Autodesk Inventor part; units mm, degrees
ref_plane "YZ Plane" through (0, 0, 0) normal (1, 0, 0) x (0, 1, 0)
ref_plane "XZ Plane" through (0, 0, 0) normal (0, 1, 0) x (-1, 0, 0)
ref_plane "XY Plane" through (0, 0, 0) normal (0, 0, 1) x (1, 0, 0)
sketch "Sketch1" plane through (0, 0, 0) normal (0, 1, 0) x (-1, 0, 0)
  line L0 (6.7628, 14.9608) -> (-5.9372, 14.9608)
  line L1 (-5.9372, 14.9608) -> (-5.9372, -112.0392)
  line L2 (-5.9372, -112.0392) -> (6.7628, -112.0392)
  line L3 (6.7628, -112.0392) -> (6.7628, 14.9608)
  point P0 (0, 0)
  dimension "d0" = 12.7
  dimension "d1" = 127
extrude "Extrusion1" add sketch "Sketch1" along normal blind 69.85
sketch "Sketch2" plane through (0, 69.85, 0) normal (0, 1, 0) x (1, 0, 0)
  line L0 (5.9372, 112.0392) -> (-6.7628, 112.0392)
  line L1 (5.9372, -14.9608) -> (5.9372, 112.0392)
  line L2 (-6.7628, -14.9608) -> (5.9372, -14.9608)
  point P0 (0, 0)
  point P1 (-0.4128, 10.4392)
  point P2 (-0.4128, 86.6392)
  dimension "d4" = 25.4
  dimension "d5" = 6.35
  dimension "d6" = 25.4
  dimension "d7" = 6.35
hole "Hole1" at (-0.4128, 69.85, -10.4392) at (-0.4128, 69.85, -86.6392) direction (0, -1, 0) diameter 4.318 end through all
sketch "Sketch3" plane through (5.9372, 0, 14.9608) normal (1, 0, 0) x (0, 0, -1)
  line L0 (0, 0) -> (0, 69.85)
  line L1 (0, 0) -> (127, 0)
  line L2 (0, 69.85) -> (127, 69.85)
  line L3 (127, 0) -> (127, 69.85)
  point P0 (14.9608, 0)
  point P1 (6.35, 57.15)
  point P2 (6.35, 12.7)
  point P3 (120.65, 57.15)
  point P4 (120.65, 12.7)
  dimension "d15" = 6.35
  dimension "d16" = 6.35
  dimension "d17" = 12.7
  dimension "d18" = 12.7
  dimension "d19" = 12.7
  dimension "d20" = 6.35
  dimension "d21" = 6.35
  dimension "d22" = 12.7
hole "Hole2" at (5.9372, 57.15, 8.6108) at (5.9372, 12.7, 8.6108) at (5.9372, 57.15, -105.6892) at (5.9372, 12.7, -105.6892) direction (-1, 0, 0) diameter 4.064 end through all counterbore diameter 9.525 counterbore depth 6.35
properties part number "BatteryFrontPlate"
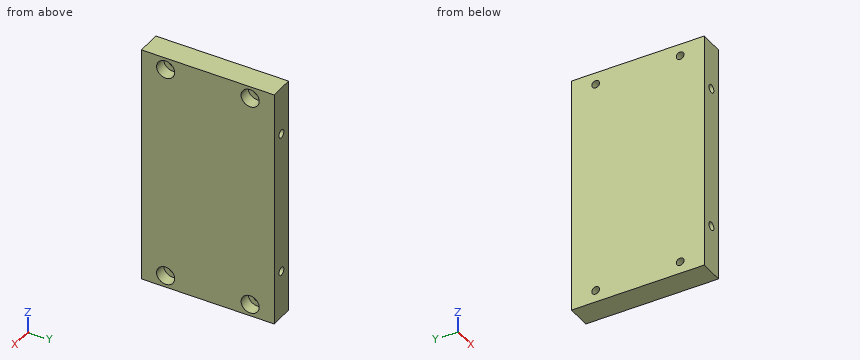
The listing builds one solid part. Answer for the finished solid, in the listing's coordinates (mm). Give positions to 0.01 mm unless a question says otherwise; leave off trailing zeros. Write each loop counter-clockwise with the first axis right and the second up, starting at its lowest first coordinate (ties: lowest second). Pieces come first, ordered by that corner, then holes. Notation, with made-up numbers: (36, 79) - (90, 79) arc R30 cw to (90, 113) - close; hole circle Ø9 at (-20.75, 29). An arc over 180 degrees is marked (long way). One line per question, with ' | ' between items. Start each with the question number.
1. Given P1, Ø3, axis at y = 12, z = -106, coming from the +X side; P2, Ø3, axis at y = 57.5, z = 8.5, coming from the +X side, each flat-ended and moving along its own axis, determine where each tip first touches the part or whether it passes through.
2. Section B-B, the plane y = 24 is taken. Determine the outline of the cut face in (x, z), then the cut area to 3 significant figures.
3. Section A-A, the plane y = 57.15 is taken. Determine the outline of the cut face in (x, z).
4. Straight lines are drawn through the part: line 1 (Z direction, x = -3.25, y = 57.15); line 2 (Y direction, x = -1.25, z = -106); line 3 (Z direction, x = 2, y = 12.7). For each, find the intervals that lie inside material, in ascending order.
Result:
1) P1: stops at x = -0.41 | P2: passes through
2) outline: (-6.76, -112.04) - (5.94, -112.04) - (5.94, 14.96) - (-6.76, 14.96) - close; hole circle Ø4.32 at (-0.41, -86.64); hole circle Ø4.32 at (-0.41, -10.44) | area: 1,580 mm2
3) outline: (-6.76, -112.04) - (5.94, -112.04) - (5.94, -110.45) - (-0.41, -110.45) - (-0.41, -107.72) - (-6.76, -107.72) - close; (-6.76, -103.66) - (-0.41, -103.66) - (-0.41, -100.93) - (5.94, -100.93) - (5.94, 3.85) - (-0.41, 3.85) - (-0.41, 6.58) - (-6.76, 6.58) - close; (-6.76, 10.64) - (-0.41, 10.64) - (-0.41, 13.37) - (5.94, 13.37) - (5.94, 14.96) - (-6.76, 14.96) - close; hole circle Ø4.32 at (-0.41, -86.64); hole circle Ø4.32 at (-0.41, -10.44)
4) line 1: z = -112.04 to -107.72, -103.66 to 6.58, 10.64 to 14.96 | line 2: y = 0 to 10.69, 14.71 to 55.14, 59.16 to 69.85 | line 3: z = -112.04 to -110.45, -100.93 to 3.85, 13.37 to 14.96
